from build123d import *

# Parameters (mm, degrees)
BOSS_EXTRUDE1_DEPTH = 1.7
SKETCH2_W           = 5.5
SKETCH2_H           = 5.3
BOSS_EXTRUDE2_DEPTH = 4


with BuildPart() as part:
    # Sketch1 → Boss-Extrude1 (new body)
    with BuildSketch(Plane(origin=(0, 0, 0), x_dir=(1, 0, 0), z_dir=(0, 1, 0))):
        with BuildLine():
            Line((-3.75, 9.1), (3.75, 9.1))
            ThreePointArc((3.75, 9.1), (5.164213562, 8.514213562), (5.75, 7.1))
            Line((5.75, 7.1), (5.75, -9.1))
            Line((5.75, -9.1), (-5.75, -9.1))
            Line((-5.75, -9.1), (-5.75, 7.1))
            ThreePointArc((-5.75, 7.1), (-5.164213562, 8.514213562), (-3.75, 9.1))
        make_face()
    extrude(amount=BOSS_EXTRUDE1_DEPTH)

    # Sketch2 → Boss-Extrude2 (add)
    with BuildSketch(Plane(origin=(0, 1.7, 0), x_dir=(1, 0, 0), z_dir=(0, 1, 0))):
        with Locations((-1.8, -0.15)):
            Rectangle(SKETCH2_W, SKETCH2_H)
    extrude(amount=BOSS_EXTRUDE2_DEPTH)


solid = part.part
The listing builds one solid part. Answer for the finished solid, in the listing's coordinates (mm). A direction names the side the tool comes from. Round coordinates to 2 decimals unless told otherwise and drop trailing zeros. Loops run counter-clockwise (first coordinate to the right, second up) from the corner with the lowest first, then second, coordinate; pieces in that order, holes last. Notation, with made-up numbers: M 62.5,27 L 84.5,27 A9 cw 84.5,41 Z; hole C 77,86 d1. An arc over 180 degrees is marked long. Return JSON: item names as keys, results as strings.
Q1. Find section B-B, the plane z = 2. Determine the outline of the cut face in (x, y), plus the area to 4 significant figures.
Results list:
{"outline": "M -5.75,0 L 5.75,0 L 5.75,1.7 L 0.95,1.7 L 0.95,5.7 L -4.55,5.7 L -4.55,1.7 L -5.75,1.7 Z", "area": "41.55 mm2"}
Q2. Find the intervals of material crossed by line 1 along Y through (x, z) = (-2.25, 7.75); line 2 along X through (y, z) = (4.7, 0.5); line 3 along Z through (x, y) = (0.5, 4.35), in increasing order. Write a range as from..to.
Results list:
{"line 1": "y = 0..1.7", "line 2": "x = -4.55..0.95", "line 3": "z = -2.5..2.8"}
Q3. Find section C-C, the plane y = 2.1. Determine the outline of the cut face in (x, z), plus the area to 4 significant figures.
Results list:
{"outline": "M -4.55,-2.5 L 0.95,-2.5 L 0.95,2.8 L -4.55,2.8 Z", "area": "29.15 mm2"}
Q4. Find section A-A, the plane x = -0.75. Determine the outline of the cut face in (y, z), plus the area to 3 significant figures.
Results list:
{"outline": "M 0,-9.1 L 1.7,-9.1 L 1.7,-2.5 L 5.7,-2.5 L 5.7,2.8 L 1.7,2.8 L 1.7,9.1 L 0,9.1 Z", "area": "52.1 mm2"}
Q5. Find section D-D, the plane x = 3.25. Determine the outline of the cut face in (y, z), plus the area to 3 significant figures.
Results list:
{"outline": "M 0,-9.1 L 1.7,-9.1 L 1.7,9.1 L 0,9.1 Z", "area": "30.9 mm2"}
Q6. Which of the six approach directions +Z, -Z, +X, -X, +Y, -Y give full straight-line access (tool end or side, diameter ignored) to faces 1 (the face through (0.95, 4, 0)), 2 (the face through (-4.55, 4, 0)), 3 (the face through (-2, 4, 2.8))?
Results list:
{"face 1": "+Z, -Z, +X, +Y", "face 2": "+Z, -Z, -X, +Y", "face 3": "+Z, +X, -X, +Y"}
Q7. Each of these flat-tipped pins is pushed along its axis until it touches: pin 1 Ø1.2 at (x, y) = (-2, 4) entering from +Z; pin 2 Ø1.2 at (x, y) = (-1.5, 3) entering from -Z; pin 3 Ø1.2 at (y, z) = (3, 0.5) entering from -X. Where does it stop, or does it pass through?
Results list:
{"pin 1": "stops at z = 2.8", "pin 2": "stops at z = -2.5", "pin 3": "stops at x = -4.55"}
